Verification items for the finished model (mm, model axes). Face numbers are marked on the shaded views. A direction names the side the tool comes from. Round coordinates to 2 decimals unless told otherwise and drop trailing zeros. Order: outer loops, then holes, each group sorted by start corner. A loop starts at its lowest first (then second) coordinate and runs counter-clockwise, first axis right, second up. Notation, with made-up numbers: M 32.25,61 L 83.25,61 A11 ccw 83.25,68 Z; hole C 9.5,29 d11. An arc over 180 degrees is marked long. Return JSON: item names as keys, results as strings. Group by question number.
from build123d import *

# Parameters (mm, degrees)
SKETCH1_W             = 40
SKETCH1_H             = 53
BOSS_EXTRUDE1_DEPTH   = 6
SKETCH16_R            = 4.5
BOSS_EXTRUDE3_DEPTH   = 2
SKETCH16_3_R          = 4.5
BOSS_EXTRUDE4_DEPTH   = 12
CUT_EXTRUDE1_DEPTH    = 4.5
F_5_4MM_DOWEL_HOLE1_D = 5.4
F_7_4MM_DOWEL_HOLE2_D = 7.4
SKETCH2_W             = 6
SKETCH2_H             = 12
BOSS_EXTRUDE2_DEPTH   = 20
F_5_4MM_DOWEL_HOLE3_D = 5.4
FILLET1_R             = 6
MIRROR2_OUTLINE_R     = 3.7
MIRROR2_DEPTH         = 6
MIRROR2_START         = 4.5
MIRROR2_2_OUTLINE_R   = 4.5
MIRROR2_2_OUTLINE_R_2 = 2.7
MIRROR2_2_DEPTH       = 13.5
MIRROR2_3_OUTLINE_R   = 4.5
MIRROR2_3_OUTLINE_R_2 = 2.7
MIRROR2_3_DEPTH       = 3.5
MIRROR2_4_DEPTH       = 1.5
MIRROR2_START_2       = -36.2
MIRROR2_5_OUTLINE_W   = 20
MIRROR2_5_OUTLINE_H   = 12
MIRROR2_5_OUTLINE_R   = 2.7
MIRROR2_5_DEPTH       = 6
MIRROR2_START_3       = -9.8
MIRROR2_6_OUTLINE_W   = 20
MIRROR2_6_OUTLINE_H   = 12
MIRROR2_6_OUTLINE_R   = 2.7
MIRROR2_6_DEPTH       = 6


# Read off the part's stored shape, not the designer's step: Mirror2
with BuildPart() as part:
    # Sketch1 → Boss-Extrude1 (new body)
    with BuildSketch(Plane(origin=(0, 0, 0), x_dir=(1, 0, 0), z_dir=(0, 1, 0))):
        with Locations((20, 26.5)):
            Rectangle(SKETCH1_W, SKETCH1_H)
    extrude(amount=BOSS_EXTRUDE1_DEPTH)

    # Sketch16 → Boss-Extrude3 (add)
    with BuildSketch(Plane(origin=(0, 6, 0), x_dir=(1, 0, 0), z_dir=(0, 1, 0))):
        with Locations(Location((16, 25, 0), (0, 0, 90))):
            Circle(SKETCH16_R)
    extrude(amount=BOSS_EXTRUDE3_DEPTH)

    # Sketch16<3> → Boss-Extrude4 (add)
    with BuildSketch(Plane(origin=(0, 6, 0), x_dir=(1, 0, 0), z_dir=(0, 1, 0))):
        with Locations(Location((24, 13, 0), (0, 0, 90))):
            Circle(SKETCH16_3_R)
    extrude(amount=BOSS_EXTRUDE4_DEPTH)

    # Sketch12 → Cut-Extrude1 (cut)
    with BuildSketch(Plane.XZ):
        Polygon((28.2, -10.575128869), (24, -8.150257739), (19.8, -10.575128869), (19.8, -15.424871131), (24, -17.849742261), (28.2, -15.424871131), align=None)
        Polygon((16, -20.150257739), (11.8, -22.575128869), (11.8, -27.424871131), (16, -29.849742261), (20.2, -27.424871131), (20.2, -22.575128869), align=None)
    extrude(amount=-CUT_EXTRUDE1_DEPTH, mode=Mode.SUBTRACT)

    # Ø5.4mm Dowel Hole1 (through all)
    with Locations(Plane(origin=(0, 0, 0), x_dir=(-1, 0, 0), z_dir=(0, -1, 0))):
        with Locations((-16, 25), (-24, 13)):
            Hole(F_5_4MM_DOWEL_HOLE1_D / 2)

    # Ø7.4mm Dowel Hole2 (through all)
    with Locations(Plane(origin=(0, 6, 0), x_dir=(1, 0, 0), z_dir=(0, 1, 0))):
        with Locations((7, 46)):
            f_7_4mm_dowel_hole2 = Hole(F_7_4MM_DOWEL_HOLE2_D / 2)

    # Sketch2 → Boss-Extrude2 (add)
    with BuildSketch(Plane.XZ):
        with Locations((6.8, -6)):
            Rectangle(SKETCH2_W, SKETCH2_H)
    boss_extrude2 = extrude(amount=BOSS_EXTRUDE2_DEPTH)

    # Ø5.4mm Dowel Hole3 (through all)
    with Locations(Plane(origin=(9.8, 0, 0), x_dir=(0, 0, -1), z_dir=(1, 0, 0))):
        with Locations((6, -10)):
            f_5_4mm_dowel_hole3 = Hole(F_5_4MM_DOWEL_HOLE3_D / 2)

    # Mirror1: Ø7.4mm Dowel Hole2, Boss-Extrude2, Ø5.4mm Dowel Hole3 across plane
    add(f_7_4mm_dowel_hole2.mirror(Plane(origin=(20, 0, 0), x_dir=(0, 0, 1), z_dir=(1, 0, 0))), mode=Mode.SUBTRACT)
    add(boss_extrude2.mirror(Plane(origin=(20, 0, 0), x_dir=(0, 0, 1), z_dir=(1, 0, 0))))
    add(f_5_4mm_dowel_hole3.mirror(Plane(origin=(20, 0, 0), x_dir=(0, 0, 1), z_dir=(1, 0, 0))), mode=Mode.SUBTRACT)

    # Fillet1
    fillet1_edges = [part.edges().sort_by_distance(p)[0] for p in [
        (0, 3, -53),
        (40, 3, -53),
    ]]
    fillet(fillet1_edges, radius=FILLET1_R)

    # Mirror2 outline → Mirror2 (add)
    with BuildSketch(Plane(origin=(0, 0, 0), x_dir=(1, 0, 0), z_dir=(0, 1, 0))):
        with BuildLine():
            Line((-6, 53), (-34, 53))
            ThreePointArc((-34, 53), (-38.242640687, 51.242640687), (-40, 47))
            Line((-40, 47), (-40, 0))
            Line((-40, 0), (0, 0))
            Line((0, 0), (0, 47))
            ThreePointArc((0, 47), (-1.757359313, 51.242640687), (-6, 53))
        make_face()
        Polygon((-19.8, 10.575128869), (-24, 8.150257739), (-28.2, 10.575128869), (-28.2, 15.424871131), (-24, 17.849742261), (-19.8, 15.424871131), align=None, mode=Mode.SUBTRACT)
        with Locations((-33, 46)):
            Circle(MIRROR2_OUTLINE_R, mode=Mode.SUBTRACT)
        with Locations((-7, 46)):
            Circle(MIRROR2_OUTLINE_R, mode=Mode.SUBTRACT)
        Polygon((-11.8, 27.424871131), (-11.8, 22.575128869), (-16, 20.150257739), (-20.2, 22.575128869), (-20.2, 27.424871131), (-16, 29.849742261), align=None, mode=Mode.SUBTRACT)
    extrude(amount=MIRROR2_DEPTH)

    # Mirror2 2 outline → Mirror2 2 (add)
    with BuildSketch(Plane(origin=(0, 0, 0), x_dir=(1, 0, 0), z_dir=(0, 1, 0)).offset(MIRROR2_START)):
        with Locations((-24, 13)):
            Circle(MIRROR2_2_OUTLINE_R)
        with Locations((-24, 13)):
            Circle(MIRROR2_2_OUTLINE_R_2, mode=Mode.SUBTRACT)
    extrude(amount=MIRROR2_2_DEPTH)

    # Mirror2 3 outline → Mirror2 3 (add)
    with BuildSketch(Plane(origin=(0, 0, 0), x_dir=(1, 0, 0), z_dir=(0, 1, 0)).offset(MIRROR2_START)):
        with Locations((-16, 25)):
            Circle(MIRROR2_3_OUTLINE_R)
        with Locations((-16, 25)):
            Circle(MIRROR2_3_OUTLINE_R_2, mode=Mode.SUBTRACT)
    extrude(amount=MIRROR2_3_DEPTH)

    # Mirror2 4 outline → Mirror2 4 (add)
    with BuildSketch(Plane(origin=(0, 0, 0), x_dir=(1, 0, 0), z_dir=(0, 1, 0)).offset(MIRROR2_START)):
        with BuildLine():
            ThreePointArc((-20.500893142, 15.829531975), (-20.102885683, 15.25), (-19.8, 14.615549442))
            Line((-19.8, 14.615549442), (-19.8, 15.424871131))
            Line((-19.8, 15.424871131), (-20.500893142, 15.829531975))
        make_face()
        with BuildLine():
            Line((-19.8, 10.575128869), (-19.8, 11.384450558))
            ThreePointArc((-19.8, 11.384450558), (-20.102885683, 10.75), (-20.500893142, 10.170468025))
            Line((-20.500893142, 10.170468025), (-19.8, 10.575128869))
        make_face()
        with BuildLine():
            ThreePointArc((-24.700893142, 17.445081417), (-24, 17.5), (-23.299106858, 17.445081417))
            Line((-23.299106858, 17.445081417), (-24, 17.849742261))
            Line((-24, 17.849742261), (-24.700893142, 17.445081417))
        make_face()
        with BuildLine():
            Line((-24, 8.150257739), (-23.299106858, 8.554918583))
            ThreePointArc((-23.299106858, 8.554918583), (-24, 8.5), (-24.700893142, 8.554918583))
            Line((-24.700893142, 8.554918583), (-24, 8.150257739))
        make_face()
        with BuildLine():
            ThreePointArc((-28.2, 14.615549442), (-27.897114317, 15.25), (-27.499106858, 15.829531975))
            Line((-27.499106858, 15.829531975), (-28.2, 15.424871131))
            Line((-28.2, 15.424871131), (-28.2, 14.615549442))
        make_face()
        with BuildLine():
            Line((-28.2, 10.575128869), (-27.499106858, 10.170468025))
            ThreePointArc((-27.499106858, 10.170468025), (-27.897114317, 10.75), (-28.2, 11.384450558))
            Line((-28.2, 11.384450558), (-28.2, 10.575128869))
        make_face()
        with BuildLine():
            ThreePointArc((-12.500893142, 27.829531975), (-12.102885683, 27.25), (-11.8, 26.615549442))
            Line((-11.8, 26.615549442), (-11.8, 27.424871131))
            Line((-11.8, 27.424871131), (-12.500893142, 27.829531975))
        make_face()
        with BuildLine():
            Line((-11.8, 22.575128869), (-11.8, 23.384450558))
            ThreePointArc((-11.8, 23.384450558), (-12.102885683, 22.75), (-12.500893142, 22.170468025))
            Line((-12.500893142, 22.170468025), (-11.8, 22.575128869))
        make_face()
        with BuildLine():
            ThreePointArc((-16.700893142, 29.445081417), (-16, 29.5), (-15.299106858, 29.445081417))
            Line((-15.299106858, 29.445081417), (-16, 29.849742261))
            Line((-16, 29.849742261), (-16.700893142, 29.445081417))
        make_face()
        with BuildLine():
            Line((-16, 20.150257739), (-15.299106858, 20.554918583))
            ThreePointArc((-15.299106858, 20.554918583), (-16, 20.5), (-16.700893142, 20.554918583))
            Line((-16.700893142, 20.554918583), (-16, 20.150257739))
        make_face()
        with BuildLine():
            ThreePointArc((-20.2, 26.615549442), (-19.897114317, 27.25), (-19.499106858, 27.829531975))
            Line((-19.499106858, 27.829531975), (-20.2, 27.424871131))
            Line((-20.2, 27.424871131), (-20.2, 26.615549442))
        make_face()
        with BuildLine():
            Line((-20.2, 22.575128869), (-19.499106858, 22.170468025))
            ThreePointArc((-19.499106858, 22.170468025), (-19.897114317, 22.75), (-20.2, 23.384450558))
            Line((-20.2, 23.384450558), (-20.2, 22.575128869))
        make_face()
    extrude(amount=MIRROR2_4_DEPTH)

    # Mirror2 5 outline → Mirror2 5 (add)
    with BuildSketch(Plane.YZ.offset(MIRROR2_START_2)):
        with Locations((-10, -6)):
            Rectangle(MIRROR2_5_OUTLINE_W, MIRROR2_5_OUTLINE_H)
        with Locations((-10, -6)):
            Circle(MIRROR2_5_OUTLINE_R, mode=Mode.SUBTRACT)
    extrude(amount=MIRROR2_5_DEPTH)

    # Mirror2 6 outline → Mirror2 6 (add)
    with BuildSketch(Plane.YZ.offset(MIRROR2_START_3)):
        with Locations((-10, -6)):
            Rectangle(MIRROR2_6_OUTLINE_W, MIRROR2_6_OUTLINE_H)
        with Locations((-10, -6)):
            Circle(MIRROR2_6_OUTLINE_R, mode=Mode.SUBTRACT)
    extrude(amount=MIRROR2_6_DEPTH)

    # Split1
    split(bisect_by=Plane(origin=(0, 0, 0), x_dir=(0, 0, 1), z_dir=(1, 0, 0)), keep=Keep.BOTTOM)


solid = part.part
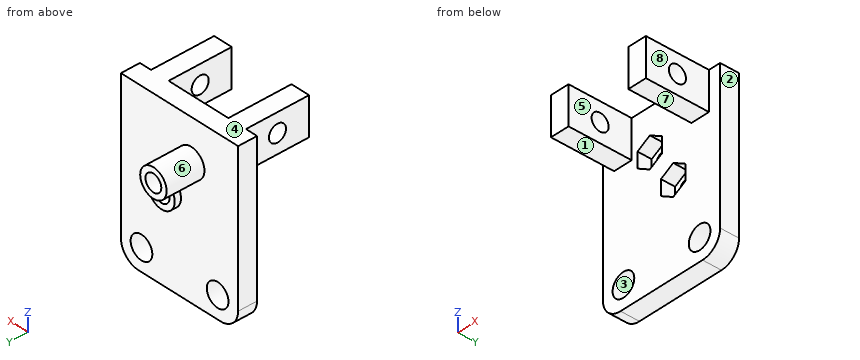
1. Cross-section at C-C (z = -46). Enter the section's corners in (x, y).
2. Access from +Z, -Z, +X, -X, +Y, -Y to the whole of each face (thin tool, end or side, straight path). Record for the marked faces 5, 6, 7 and 8.
3. Draft check along Z on the marked faces 1, 2, 3 and 4. Enter one of: +Z half, -Z half, draft (parallel to the pull), parting line (faces both ways), or undercut.
4. Cross-section at A-A (x = -7). Enter the section's corners in (y, z).
5. Cross-section at B-B (y = -10). Enter the section's corners in (x, z), plus the area to 3 significant figures.
6. Thickness scan on line 1 along X through (y, z) = (3.6, -46); line 2 along X through (y, z) = (5.9, -25); line 3 along X through (y, z) = (2.5, -15). Record the ranges inside material, lowest first. Write a range as from..to.
7. Cross-section at D-D (z = -13). Enter the section's corners in (x, y).
8. Go/stop test with flat-tipped pins: pin 1 (6 mm diameter, centred on x = -16, z = -25, fed in from +Y); pin 2 (6 mm diameter, centred on x = -19.5, z = -11, fed in from +Y); pin 3 (10 mm diameter, centred on x = -5, z = -18, fed in from -Y); pin 4 (3 mm diameter, centred on y = -12.5, z = -8, fed in from -X). Record where each tip stops, or that it passes through.
Computed:
{
 "1": {"outline": "M -40,0 L -36.7,0 L -36.7,6 L -40,6 Z; M -29.3,0 L -10.7,0 L -10.7,6 L -29.3,6 Z; M -3.3,0 L 0,0 L 0,6 L -3.3,6 Z"},
 "2": {"face 5": "+Z, -Z, -Y", "face 6": "+Y", "face 7": "-Z, +X, -X, -Y", "face 8": "+Z, -Z, +X, -Y"},
 "3": {"face 1": "-Z half", "face 2": "draft", "face 3": "undercut", "face 4": "+Z half"},
 "4": {"outline": "M -20,-12 L 0,-12 L 0,-42.3 L 6,-42.3 L 6,0 L -20,0 Z; M 0,-53 L 6,-53 L 6,-49.7 L 0,-49.7 Z; hole C -10,-6 d5.4"},
 "5": {"outline": "M -36.2,-12 L -30.2,-12 L -30.2,-8.7 L -36.2,-8.7 Z; M -36.2,-3.3 L -30.2,-3.3 L -30.2,0 L -36.2,0 Z; M -9.8,-12 L -3.8,-12 L -3.8,-8.7 L -9.8,-8.7 Z; M -9.8,-3.3 L -3.8,-3.3 L -3.8,0 L -9.8,0 Z", "area": "79.2 mm²"},
 "6": {"line 1": "x = -40..-36.7, -29.3..-10.7, -3.3..0", "line 2": "x = -40..-18.7, -13.3..0", "line 3": "x = -40..-28.2, -19.8..0"},
 "7": {"outline": "M -40,0 L -28.2,0 L -28.2,4.5 L -26.7,4.5 L -26.7,18 L -28.5,18 L -28.5,6 L -40,6 Z; M -21.3,4.5 L -19.8,4.5 L -19.8,0 L 0,0 L 0,6 L -19.5,6 L -19.5,18 L -21.3,18 Z"},
 "8": {"pin 1": "stops at y = 8", "pin 2": "stops at y = 18", "pin 3": "stops at y = 0", "pin 4": "stops at x = -36.2"}
}
